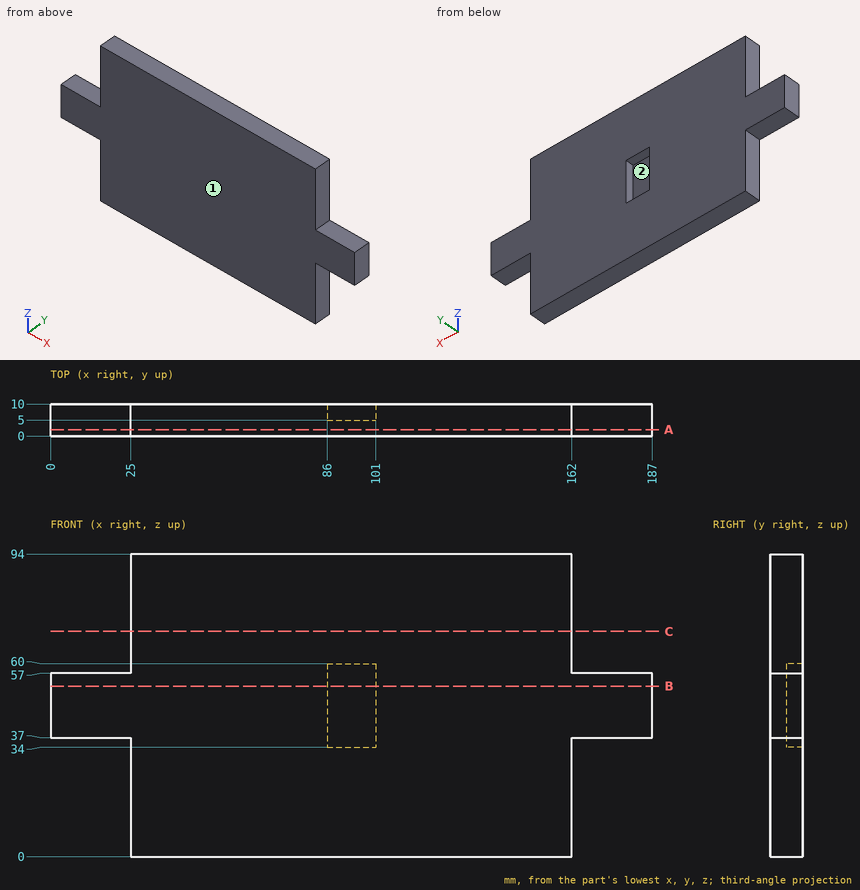
The drawing under review shows one solid part. Ordinate dimensions are in mm from its lowest x, y, z. Round coordinates to 2 decimals unless told otherwise and drop trailing zeros. Write each loop counter-clockwise with the first axis right and the second up, starting at its lowest first coordinate (ties: lowest second). Pieces come first, ordered by that corner, then holes. Notation, with made-up numbers: (-15, 87) - (27, 87) arc R16 cw to (27, 118) - close; hole circle Ø3 at (-36, 14.5). An arc over 180 degrees is marked (long way). Use a Markdown table: item, result. Add a question column.
1. We need section C-C (z = 70). State the section outline as (x, y) points, then the cut area to 3 significant figures.
2. Mouldability with a two-part tool opening along Z and no side actions: class the marked faces 1 and 2 as +Z half, -Z half, draft (parallel to the pull), parting line (faces both ways), or undercut.
3. Wall thickness on probe 1 along Z at (x, y) = (92.5, 9); probe 2 along X at (y, z) = (7, 75.5); probe 3 along Z at (x, y) = (22, 8.5): over which ranges is each line inside the solid? List them lowest first.
4. Clearance check with flat-ended pins moving along their axes: pin 1 (5 mm diameter, centred on y = 3, z = 20, fed in from -X); pin 2 (7.5 mm diameter, centred on x = 92.5, z = 45, fed in from +Y); pin 3 (3 mm diameter, centred on y = 4.5, z = 76.5, fed in from +X). State where each tip first meets the part, or that it passes through.
5. We need section A-A (y = 2). State the section outline as (x, z) points, then the cut area to 3 significant figures.
6. We need section B-B (z = 53). State the section outline as (x, y) points, then the cut area to 4 significant figures.
Output:
| question | item | result |
|---|---|---|
| 1 | outline | (25, 0) - (162, 0) - (162, 10) - (25, 10) - close |
| 1 | area | 1,370 mm2 |
| 2 | face 1 | draft |
| 2 | face 2 | undercut |
| 3 | probe 1 | z = 0 to 34, 60 to 94 |
| 3 | probe 2 | x = 25 to 162 |
| 3 | probe 3 | z = 37 to 57 |
| 4 | pin 1 | stops at x = 25 |
| 4 | pin 2 | stops at y = 5 |
| 4 | pin 3 | stops at x = 162 |
| 5 | outline | (0, 37) - (25, 37) - (25, 0) - (162, 0) - (162, 37) - (187, 37) - (187, 57) - (162, 57) - (162, 94) - (25, 94) - (25, 57) - (0, 57) - close |
| 5 | area | 13,900 mm2 |
| 6 | outline | (0, 0) - (187, 0) - (187, 10) - (101, 10) - (101, 5) - (86, 5) - (86, 10) - (0, 10) - close |
| 6 | area | 1,795 mm2 |
